Read the model definition and answer for the solid it produces. Units are mm, in the model's axes. Face numbers are marked on the shaded views. A direction names the side the tool comes from. Round coordinates to 2 decimals unless told otherwise and drop trailing zeros. Loops run counter-clockwise (first coordinate to the right, second up) from the corner with the lowest first, then second, coordinate; pieces in that order, holes last. Notation, with made-up numbers: (30, 19.5) - (64, 19.5) arc R31 ccw to (64, 46.5) - close; hole circle Ø4 at (81.25, 83.25). An arc over 180 degrees is marked (long way). Answer as CSV lines item,"result".
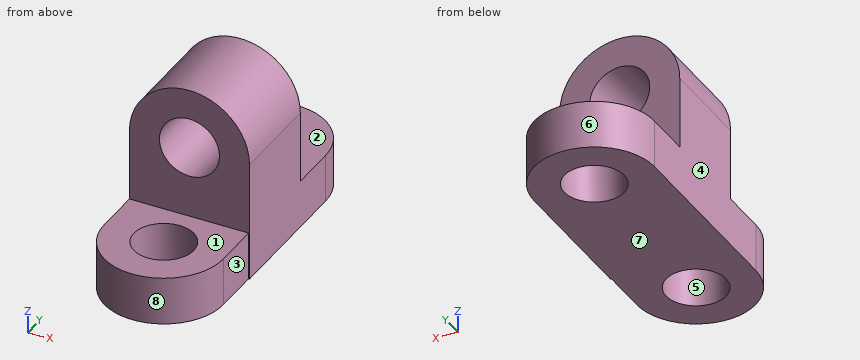
```python
from build123d import *

# Parameters (mm, degrees)
F1_DEPTH = 40
F3_DEPTH = 20
F5_DEPTH = 20


with BuildPart() as f1:
    # F0 (on Front) → F1 (new body)
    with BuildSketch(Plane.XZ):
        with BuildLine():
            Line((0, 50), (0, 0))
            Line((0, 0), (50, 0))
            Line((50, 0), (50, 50))
            Line((50, 50), (37.5, 50))
            ThreePointArc((37.5, 50), (25, 37.5), (12.5, 50))
            Line((12.5, 50), (0, 50))
        make_face()
        with BuildLine():
            ThreePointArc((50, 50), (25, 75), (0, 50))
            Line((0, 50), (12.5, 50))
            ThreePointArc((12.5, 50), (25, 62.5), (37.5, 50))
            Line((37.5, 50), (50, 50))
        make_face()
    extrude(amount=F1_DEPTH)

    # F2 (on Top) → F3 (join)
    with BuildSketch(Plane.XY):
        with BuildLine():
            Line((0, 20), (0, 0))
            Line((0, 0), (50, 0))
            Line((50, 0), (50, 20))
            Line((50, 20), (37.5, 20))
            ThreePointArc((37.5, 20), (25, 7.5), (12.5, 20))
            Line((12.5, 20), (0, 20))
        make_face()
        with BuildLine():
            ThreePointArc((50, 20), (25, 45), (0, 20))
            Line((0, 20), (12.5, 20))
            ThreePointArc((12.5, 20), (25, 32.5), (37.5, 20))
            Line((37.5, 20), (50, 20))
        make_face()
    extrude(amount=F3_DEPTH)

    # F4 (on Top) → F5 (join)
    with BuildSketch(Plane.XY):
        with BuildLine():
            Line((49.637856, -39.829515), (0, -39.829515))
            Line((0, -39.829515), (0, -59.829515))
            Line((0, -59.829515), (12.318928, -59.829515))
            ThreePointArc((12.318928, -59.829515), (24.818928, -47.329515), (37.318928, -59.829515))
            Line((37.318928, -59.829515), (49.637856, -59.829515))
            Line((49.637856, -59.829515), (49.637856, -39.829515))
        make_face()
        with BuildLine():
            Line((12.318928, -59.829515), (0, -59.829515))
            ThreePointArc((0, -59.829515), (24.818928, -84.648443), (49.637856, -59.829515))
            Line((49.637856, -59.829515), (37.318928, -59.829515))
            ThreePointArc((37.318928, -59.829515), (24.818928, -72.329515), (12.318928, -59.829515))
        make_face()
    extrude(amount=F5_DEPTH)


solid = f1.part
```
1) Each of these flat-tipped pins is pushed along its axis until it touches: P1, Ø6, axis at x = 39, z = 35.5, coming from the +Y side; P2, Ø22.5, axis at x = 23, y = -66, coming from the +Z side; P3, Ø10, axis at y = -50, z = 6.5, coming from the +X side. Where does it stop, or does it pass through?
Entries:
P1,"stops at y = 0"
P2,"stops at z = 20"
P3,"stops at x = 49.64"
2) Find the intervals of material crossed by line 1 (Y direction, x = 25, z = 11.5); line 2 (Z direction, x = 25, y = -12.5); line 3 (X direction, y = 21, z = 16), in increasing order.
Entries:
line 1,"y = -84.65 to -72.33, -47.33 to 7.5, 32.5 to 45"
line 2,"z = 0 to 37.5, 62.5 to 75"
line 3,"x = 0.02 to 12.54, 37.46 to 49.98"
3) A cutting plane is placed at C-C, the plane z = 39. Determine the outline of the cut face in (x, y), plus the area to 3 significant figures.
Entries:
outline,"(0, -40) - (19.06, -40) - (19.06, 0) - (0, 0) - close; (30.94, -40) - (50, -40) - (50, 0) - (30.94, 0) - close"
area,"1,530 mm^2"
4) A cutting plane is placed at B-B, the plane x = 23. Determine the outline of the cut face in (y, z).
Entries:
outline,"(-84.58, 0) - (-72.2, 0) - (-72.2, 20) - (-84.58, 20) - close; (-47.46, 0) - (7.66, 0) - (7.66, 20) - (0, 20) - (0, 37.66) - (-40, 37.66) - (-40, 20) - (-47.46, 20) - close; (-40, 62.34) - (0, 62.34) - (0, 74.92) - (-40, 74.92) - close; (32.34, 0) - (44.92, 0) - (44.92, 20) - (32.34, 20) - close"
5) A tool of negligible diameter and unlimited length cuts with its end or side. For the marked faces 1, 2, 3 and 4, from which of +Z, -Z, +X, -X, +Y, -Y can it reach the whole face along a straight path? Write none if from no direction.
Entries:
face 1,"+Z, +X, -X, -Y"
face 2,"+Z, +X, -X, +Y"
face 3,"+Z, -Z, +X, -Y"
face 4,"+Z, -Z, -X, +Y, -Y"
6) A cutting plane is placed at A-A, the plane y = 21.5. Determine the outline of the cut face in (x, z), plus the area to 3 significant figures.
Entries:
outline,"(0.05, 0) - (12.59, 0) - (12.59, 20) - (0.05, 20) - close; (37.41, 0) - (49.95, 0) - (49.95, 20) - (37.41, 20) - close"
area,"502 mm^2"
7) The mould has two halves that part along Y. Classify the marked faces 5, 6, 7 and 8: pulls with the +Y half, pulls with the -Y half, needs draft (parallel to the pull), parting line crosses it, or undercut.
Entries:
face 5,"undercut"
face 6,"pulls with the +Y half"
face 7,"needs draft"
face 8,"pulls with the -Y half"
8) A cutting plane is placed at D-D, the plane x = 45.5. Determine the outline of the cut face in (y, z).
Entries:
outline,"(-73.55, 0) - (34.31, 0) - (34.31, 20) - (0, 20) - (0, 64.31) - (-40, 64.31) - (-40, 20) - (-73.55, 20) - close"
